from build123d import *

# Parameters (mm, degrees)
SKETCH_1_W           = 94
SKETCH_1_H           = 26
EXTRUDE_1_DEPTH      = 21.2
SKETCH_1_7_R         = 0.7
CUT_EXTRUDE_1_DEPTH  = 3
SKETCH_2_W           = 77.9
SKETCH_2_H           = 21.4
CUT_EXTRUDE_2_DEPTH  = 19.3
SKETCH_5_W           = 5.5
SKETCH_5_H           = 8
CUT_EXTRUDE_3_DEPTH  = 2
SKETCH_6_W           = 76
SKETCH_6_H           = 24
CUT_EXTRUDE_4_DEPTH  = 3
SKETCH_7_R           = 10.15
SKETCH_7_W           = 10
SKETCH_7_H           = 1.516965414
CUT_EXTRUDE_5_DEPTH  = 2
SKETCH_8_R           = 8
CUT_EXTRUDE_6_DEPTH  = 4
CUT_EXTRUDE_12_DEPTH = 2
SKETCH_10_R          = 0.6
CUT_EXTRUDE_13_DEPTH = 3
CUT_EXTRUDE_START    = -23
SKETCH_10_3_R        = 0.6
CUT_EXTRUDE_14_DEPTH = 3
SKETCH_11_W          = 2.5
SKETCH_11_H          = 11
CUT_EXTRUDE_15_DEPTH = 3
SKETCH_12_R          = 0.3
CUT_EXTRUDE_16_DEPTH = 3
SKETCH_13_W          = 12
SKETCH_13_H          = 3
CUT_EXTRUDE_17_DEPTH = 11


with BuildPart() as part:
    # 草图1 → 凸台-拉伸1 (new body)
    with BuildSketch(Plane(origin=(0, 0, 0), x_dir=(1, 0, 0), z_dir=(0, 1, 0))):
        Rectangle(SKETCH_1_W, SKETCH_1_H)
    extrude(amount=EXTRUDE_1_DEPTH)

    # 草图1<7> → 切除-拉伸1 (cut)
    with BuildSketch(Plane(origin=(0, 0, 0), x_dir=(1, 0, 0), z_dir=(0, 1, 0))):
        with Locations(Location((-44, 10, 0), (0, 0, 270))):
            Circle(SKETCH_1_7_R)
        with Locations(Location((-44, -10, 0), (0, 0, 270))):
            Circle(SKETCH_1_7_R)
        with Locations(Location((44, 10, 0), (0, 0, 270))):
            Circle(SKETCH_1_7_R)
        with Locations(Location((44, -10, 0), (0, 0, 270))):
            Circle(SKETCH_1_7_R)
    extrude(amount=CUT_EXTRUDE_1_DEPTH, mode=Mode.SUBTRACT)

    # 草图2 → 切除-拉伸2 (cut)
    with BuildSketch(Plane.XZ):
        with Locations((1.95, 0)):
            Rectangle(SKETCH_2_W, SKETCH_2_H)
    extrude(amount=-CUT_EXTRUDE_2_DEPTH, mode=Mode.SUBTRACT)

    # 草图5 → 切除-拉伸3 (cut)
    with BuildSketch(Plane.XZ):
        with Locations((-39.75, 0)):
            Rectangle(SKETCH_5_W, SKETCH_5_H)
        with Locations((43.65, 0)):
            Rectangle(SKETCH_5_W, SKETCH_5_H)
    extrude(amount=-CUT_EXTRUDE_3_DEPTH, mode=Mode.SUBTRACT)

    # 草图6 → 切除-拉伸4 (cut)
    with BuildSketch(Plane.XZ):
        with Locations((2, 0)):
            Rectangle(SKETCH_6_W, SKETCH_6_H)
    extrude(amount=-CUT_EXTRUDE_4_DEPTH, mode=Mode.SUBTRACT)

    # 草图7 → 切除-拉伸5 (cut)
    with BuildSketch(Plane(origin=(47, 0, 0), x_dir=(0, 0, -1), z_dir=(1, 0, 0))):
        with Locations((0, 10.35)):
            Circle(SKETCH_7_R)
        with Locations((0, 0.758482707)):
            Rectangle(SKETCH_7_W, SKETCH_7_H)
    extrude(amount=-CUT_EXTRUDE_5_DEPTH, mode=Mode.SUBTRACT)

    # 草图8 → 切除-拉伸6 (cut)
    with BuildSketch(Plane(origin=(45, 0, 0), x_dir=(0, 0, -1), z_dir=(1, 0, 0))):
        with Locations((0, 10.35)):
            Circle(SKETCH_8_R)
    extrude(amount=-CUT_EXTRUDE_6_DEPTH, mode=Mode.SUBTRACT)

    # 草图9 → 切除-拉伸12 (cut)
    with BuildSketch(Plane(origin=(47, 0, 0), x_dir=(0, 0, -1), z_dir=(1, 0, 0))):
        with BuildLine():
            Line((-7.775351098, 16.874294238), (0, 10.35))
            Line((0, 10.35), (7.775351098, 16.874294238))
            ThreePointArc((7.775351098, 16.874294238), (0, 20.5), (-7.775351098, 16.874294238))
        make_face()
        with BuildLine():
            ThreePointArc((-7.775351098, 16.874294238), (0, 20.5), (7.775351098, 16.874294238))
            Line((7.775351098, 16.874294238), (11.107644425, 19.67042034))
            ThreePointArc((11.107644425, 19.67042034), (10.391564404, 20.462635128), (9.619121582, 21.2))
            Line((9.619121582, 21.2), (-9.619121582, 21.2))
            ThreePointArc((-9.619121582, 21.2), (-10.391564404, 20.462635128), (-11.107644425, 19.67042034))
            Line((-11.107644425, 19.67042034), (-7.775351098, 16.874294238))
        make_face()
    extrude(amount=-CUT_EXTRUDE_12_DEPTH, mode=Mode.SUBTRACT)

    # 草图10 → 切除-拉伸13 (cut)
    with BuildSketch(Plane(origin=(0, 0, -13), x_dir=(-1, 0, 0), z_dir=(0, 0, -1))):
        with Locations((-43, 18.2)):
            Circle(SKETCH_10_R)
        with Locations((-43, 3)):
            Circle(SKETCH_10_R)
    extrude(amount=-CUT_EXTRUDE_13_DEPTH, mode=Mode.SUBTRACT)

    # 草图10<3> → 切除-拉伸14 (cut)
    with BuildSketch(Plane(origin=(0, 0, -13), x_dir=(-1, 0, 0), z_dir=(0, 0, -1)).offset(CUT_EXTRUDE_START)):
        with Locations((-43, 18.2)):
            Circle(SKETCH_10_3_R)
        with Locations((-43, 3)):
            Circle(SKETCH_10_3_R)
    extrude(amount=-CUT_EXTRUDE_14_DEPTH, mode=Mode.SUBTRACT)

    # 草图11 → 切除-拉伸15 (cut)
    with BuildSketch(Plane.XZ):
        with Locations((-44.7, 2.65)):
            Rectangle(SKETCH_11_W, SKETCH_11_H)
    extrude(amount=-CUT_EXTRUDE_15_DEPTH, mode=Mode.SUBTRACT)

    # 草图12 → 切除-拉伸16 (cut)
    with BuildSketch(Plane.ZY.offset(47)):
        with Locations((-8.05, 2)):
            Circle(SKETCH_12_R)
        with Locations((8.05, 2)):
            Circle(SKETCH_12_R)
    extrude(amount=-CUT_EXTRUDE_16_DEPTH, mode=Mode.SUBTRACT)

    # 草图13 → 切除-拉伸17 (cut)
    with BuildSketch(Plane.ZY.offset(47)):
        with Locations((0, 1.5)):
            Rectangle(SKETCH_13_W, SKETCH_13_H)
    extrude(amount=-CUT_EXTRUDE_17_DEPTH, mode=Mode.SUBTRACT)


solid = part.part
The listing builds one solid part. Answer for the finished solid, in the listing's coordinates (mm). A direction names the side the tool comes from. Round coordinates to 2 decimals unless told otherwise and drop trailing zeros. Order: outer loops, then holes, each group sorted by start corner. A loop starts at its lowest first (then second) coordinate and runs counter-clockwise, first axis right, second up. Notation, with made-up numbers: (49.5, 57) -> (100.5, 57) arc R19 ccw to (100.5, 92) -> close; hole circle Ø3 at (12, 2). An arc over 180 degrees is marked (long way). One line per item, written item: value.
Item 1: Straight lines are drawn through the part: L1, parallel to Z at x = 44, y = 1.35; L2, parallel to X at y = 2, z = 10; L3, parallel to Z at x = -6, y = 8.75. For each, find the intervals that lie inside material, in ascending order.
Taken from the geometry:
L1: z = -13 to -10.7, -9.3 to -4, 4 to 9.3, 10.7 to 13
L2: x = -47 to -44.7, -43.3 to -37, 40.9 to 43.3, 44.7 to 47
L3: z = -13 to -10.7, 10.7 to 13
Item 2: For a pull along Z with two mould halves and no side action, classify faces 5 (the flat face through (46, 1, -5)), 6 (the flat face through (47, 8, -11)), 7 (the flat face through (-1, 10, 13)) as released by +Z, released by -Z, zero draft, split by the parting line, or undercut.
Taken from the geometry:
face 5: undercut
face 6: zero draft
face 7: released by +Z
Item 3: Find section B-B, the plane x = 21. Give the vertices of the cut face in (y, z).
Taken from the geometry:
outline: (0, -13) -> (21.2, -13) -> (21.2, 13) -> (0, 13) -> (0, 12) -> (3, 12) -> (3, 10.7) -> (19.3, 10.7) -> (19.3, -10.7) -> (3, -10.7) -> (3, -12) -> (0, -12) -> close
Item 4: Find section C-C, the plane z = 2.5. Give the vertices of the cut face in (x, y).
Taken from the geometry:
outline: (-47, 3) -> (-37, 3) -> (-37, 19.3) -> (40.9, 19.3) -> (40.9, 2) -> (45, 2) -> (45, 2.75) -> (41, 2.75) -> (41, 17.95) -> (45, 17.95) -> (45, 21.2) -> (-47, 21.2) -> close
Item 5: Given P1, Ø0.7, axis at x = 44, z = -10, coming from the -Y side; P2, Ø1, axis at x = 43, y = 3, coming from the +Z side; P3, Ø1, axis at x = 30.5, z = -8.5, coming from the -Y side, each flat-ended and moving along its own axis, determine where each tip first touches the part or whether it passes through.
Taken from the geometry:
P1: stops at y = 3
P2: stops at z = 10
P3: stops at y = 19.3
Item 6: For faces 1 (the flat face through (-42, 1, -6)), 2 (the flat face through (-37, 10, 0)), 3 (the cylindrical face through (46.014, 8.422, -9.965)), 4 (the flat face through (46, 1, 5)), determine the directions among +Z, -Z, +X, -X, +Y, -Y from which every point of the face is accessible in a straight line to the end or side of a thin tool.
Taken from the geometry:
face 1: -X, -Y
face 2: -Y
face 3: +X
face 4: +X, +Y, -Y
Item 7: Find section D-D, the plane y = 6.75. Give the vertices of the cut face in (x, z).
Taken from the geometry:
outline: (-47, -13) -> (47, -13) -> (47, -9.49) -> (45, -9.49) -> (45, -7.14) -> (41, -7.14) -> (41, 7.14) -> (45, 7.14) -> (45, 9.49) -> (47, 9.49) -> (47, 13) -> (-47, 13) -> close; hole (-37, -10.7) -> (40.9, -10.7) -> (40.9, 10.7) -> (-37, 10.7) -> close
Item 8: Find section A-A, the plane y = 10.35. Give the vertices of the cut face in (x, z).
Taken from the geometry:
outline: (-47, -13) -> (47, -13) -> (47, -10.15) -> (45, -10.15) -> (45, -8) -> (41, -8) -> (41, 8) -> (45, 8) -> (45, 10.15) -> (47, 10.15) -> (47, 13) -> (-47, 13) -> close; hole (-37, -10.7) -> (40.9, -10.7) -> (40.9, 10.7) -> (-37, 10.7) -> close
